Drawing for the job (mm, zero at the part's lowest x, y, z). A direction names the side the tool comes from. Round coordinates to 2 decimals unless told otherwise and drop trailing zeros. Loops run counter-clockwise (first coordinate to the right, second up) from the corner with the lowest first, then second, coordinate; pieces in that order, holes last. Notation, with made-up numbers: M -25.5,46.5 L 13.5,46.5 A34 ccw 13.5,84.5 Z; hole C -40,-25 d7. An arc over 180 degrees is marked long. Answer in a Markdown table with one row per item.
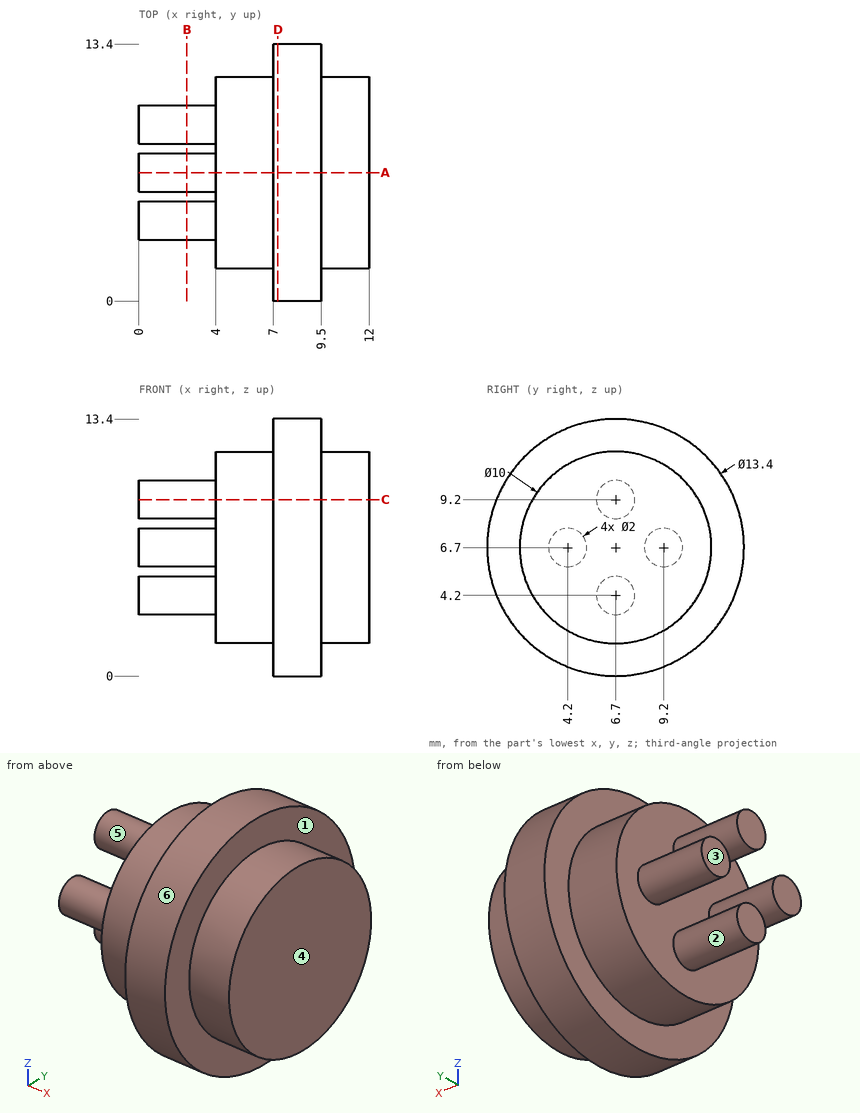
1. Saw through at A-A (y = 6.7). Write the cut outline in (x, z), and give its area (4 significant figures).
Verdict:
| item | result |
|---|---|
| outline | M 0,3.2 L 4,3.2 L 4,1.7 L 7,1.7 L 7,0 L 9.5,0 L 9.5,1.7 L 12,1.7 L 12,11.7 L 9.5,11.7 L 9.5,13.4 L 7,13.4 L 7,11.7 L 4,11.7 L 4,10.2 L 0,10.2 L 0,8.2 L 4,8.2 L 4,5.2 L 0,5.2 Z |
| area | 104.5 mm² |
2. Saw through at C-C (z = 9.2). Write the cut outline in (x, y).
Verdict:
| item | result |
|---|---|
| outline | M 0,5.7 L 4,5.7 L 4,2.37 L 7,2.37 L 7,0.48 L 9.5,0.48 L 9.5,2.37 L 12,2.37 L 12,11.03 L 9.5,11.03 L 9.5,12.92 L 7,12.92 L 7,11.03 L 4,11.03 L 4,7.7 L 0,7.7 Z |
3. Tool access for the marked faces 1, 2 and 3: list every direction of +Z, -Z, +X, -X, +Y, -Y with a clear straight run to the whole face (end or side of a thin tool).
Verdict:
| item | result |
|---|---|
| face 1 | +X |
| face 2 | -X |
| face 3 | +Z, -Z, -X, +Y, -Y |
4. Pin check, flat tips, straight feed: pin 1 (5 mm diameter, centred on x = 2.5, y = 4, fed in from -Z); pin 2 (5 mm diameter, centred on y = 4.5, z = 7.5, fed in from -X); pin 3 (1 mm diameter, centred on x = 1.5, y = 8, fed in from +Z); pin 4 (1 mm diameter, centred on x = 9, z = 8, fed in from -Y). Stop position of each tip, or through.
Verdict:
| item | result |
|---|---|
| pin 1 | stops at z = 1.75 |
| pin 2 | stops at x = 0 |
| pin 3 | stops at z = 9.8 |
| pin 4 | stops at y = 0.05 |
5. Wall check: probe 1 along X at (y, z) = (10.25, 8); probe 2 along X at (y, z) = (10.75, 11.5); probe 3 along Z at (x, y) = (7.75, 7.25). Give the ranges that are in metal, low to high.
Verdict:
| item | result |
|---|---|
| probe 1 | x = 4 to 12 |
| probe 2 | x = 7 to 9.5 |
| probe 3 | z = 0.02 to 13.38 |
6. Mould opens along Z. For the marked faces 4, 5 and 6 say: +Z half, -Z half, draft (parallel to the pull), parting line (faces both ways), or undercut.
Verdict:
| item | result |
|---|---|
| face 4 | draft |
| face 5 | undercut |
| face 6 | parting line |
7. Saw through at D-D (x = 7.25). Write the cut outline in (y, z).
Verdict:
| item | result |
|---|---|
| outline | C 6.7,6.7 d13.4 |
8. Saw through at B-B (x = 2.5). Write the cut outline in (y, z).
Verdict:
| item | result |
|---|---|
| outline | C 4.2,6.7 d2; C 6.7,4.2 d2; C 6.7,9.2 d2; C 9.2,6.7 d2 |
